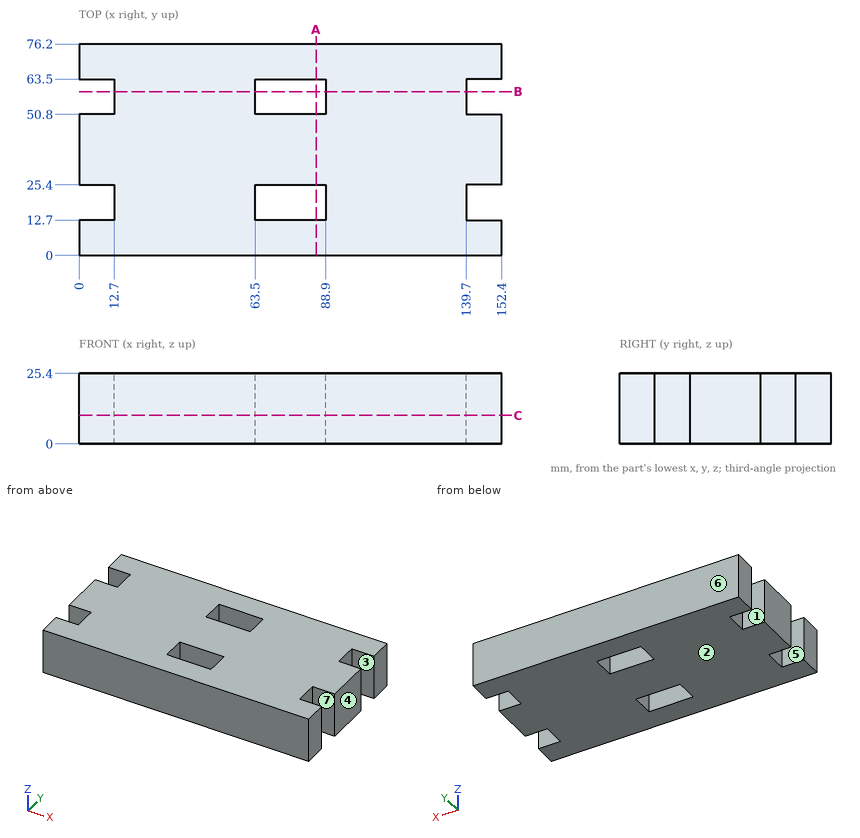
Geometry: see drawing. Coordinates: mm, zero at the bounding-box minimum. A direction names the side the tool comes from. Give positions to 0.01 mm unless a question says otherwise; leave off trailing zeros. Loops run counter-clockwise (first coordinate to the right, second up) from the corner with the lowest first, then second, coordinate; pieces in that order, holes last. Notation, with made-up numbers: (-0.75, 35) -> (31.25, 35) arc R17 cw to (31.25, 58) -> close; hole circle Ø2 at (57.5, 89). An arc over 180 degrees is marked (long way). Put each result on its own line as item: value.
1. Cut plane C-C (z = 10.25). Return the cut outline in (x, y), plus the area to 3 significant figures.
Taken from the geometry:
outline: (0, 0) -> (152.4, 0) -> (152.4, 12.7) -> (139.7, 12.7) -> (139.7, 25.4) -> (152.4, 25.4) -> (152.4, 50.8) -> (139.7, 50.8) -> (139.7, 63.5) -> (152.4, 63.5) -> (152.4, 76.2) -> (0, 76.2) -> (0, 63.5) -> (12.7, 63.5) -> (12.7, 50.8) -> (0, 50.8) -> (0, 25.4) -> (12.7, 25.4) -> (12.7, 12.7) -> (0, 12.7) -> close; hole (63.5, 12.7) -> (88.9, 12.7) -> (88.9, 25.4) -> (63.5, 25.4) -> close; hole (63.5, 50.8) -> (88.9, 50.8) -> (88.9, 63.5) -> (63.5, 63.5) -> close
area: 10,300 mm2
2. Ray query, line 1 along Y through (x, z) = (146, 22); line 2 along X through (y, z) = (13.5, 2.5). Return the intervals inside material, ascending. Write a range as [from, to].
Taken from the geometry:
line 1: y = [0, 12.7], [25.4, 50.8], [63.5, 76.2]
line 2: x = [12.7, 63.5], [88.9, 139.7]
3. Cut plane A-A (x = 85.5). Return the cut outline in (y, z).
Taken from the geometry:
outline: (0, 0) -> (12.7, 0) -> (12.7, 25.4) -> (0, 25.4) -> close; (25.4, 0) -> (50.8, 0) -> (50.8, 25.4) -> (25.4, 25.4) -> close; (63.5, 0) -> (76.2, 0) -> (76.2, 25.4) -> (63.5, 25.4) -> close
4. Set-up query: the marked faces 1, 2 and 3. Return all of +Z, -Z, +X, -X, +Y, -Y with unobstructed straight access to the full face (end or side cutting, diameter ignored); none if empty.
Taken from the geometry:
face 1: +Z, -Z, -X
face 2: -Z, +X, -X, +Y, -Y
face 3: +Z, -Z, +X
5. Pin query (flat end, axial travel): P1, Ø4, axis at y = 18, z = 7, coming from the -X side; P2, Ø12.5, axis at x = 81, z = 17.5, coming from the -Y side; P3, Ø4, axis at y = 17, z = 9.5, coming from the +X side. Return the tip coordinate at first contact, or that it passes through.
Taken from the geometry:
P1: stops at x = 12.7
P2: stops at y = 0
P3: stops at x = 139.7
6. Cut plane B-B (y = 59). Return the cut outline in (x, z).
Taken from the geometry:
outline: (12.7, 0) -> (63.5, 0) -> (63.5, 25.4) -> (12.7, 25.4) -> close; (88.9, 0) -> (139.7, 0) -> (139.7, 25.4) -> (88.9, 25.4) -> close
7. Pull-direction query (Y, two-part tool) for the marked faces 4, 5, 6 and 7; classes: released by +Y, released by -Y, zero draft, split by the parting line, or undercut.
Taken from the geometry:
face 4: zero draft
face 5: undercut
face 6: released by +Y
face 7: undercut
